Autodesk Fusion 360 part; units mm, degrees
sketch "Sketch1" plane through (0, 0, 0) normal (0, 0, 1) x (1, 0, 0)
  circle A0 centre (0, 0) radius 5
  circle A1 centre (0, 0) radius 2.5
  dimension "d1" = 10
  dimension "d2" = 5
extrude "Extrude1" add sketch "Sketch1" along normal blind 10
sketch "Sketch2" plane through (0, 0, 10) normal (0, 0, 1) x (-1, 0, 0)
  circle A0 centre (0, 0) radius 2.5
  circle A1 centre (0, 0) radius 5
  line L0 (0, 0) -> (-5.75, 0)
  line L1 (-5.75, 0) -> (-5.75, -5.75)
  line L2 (-5.75, -5.75) -> (5.75, -5.75)
  line L3 (5.75, -5.75) -> (5.75, 5.75)
  line L4 (5.75, 5.75) -> (-5.75, 5.75)
  line L5 (-5.75, 5.75) -> (-5.75, -5.75)
  dimension "d5" = 5.75
  dimension "d6" = 5.75
  dimension "d7" = 11.5
  dimension "d8" = 11.5
extrude "Extrude2" add sketch "Sketch2" along normal blind 13 contours A0 | A1 | L1 L2 L3 L4 L5
fillet "Fillet1" radius 5.75 2 edges at (0, -5.75, 23) (0, 5.75, 23)
hole "Hole1" at (5.75, 0, 17.25) direction (-1, 0, 0) diameter 4 depth 11.5 tip angle 180
equation "d5 = ( 11.5 / 2 ) * 1 mm"
Geometry: final body of the model. Coordinates: model frame, mm. A direction names the side the tool comes from. Coordinates: 2 decimals unless noted, no trailing zeros. Order: outer loops, then holes, each group sorted by start corner. A loop starts at its lowest first (then second) coordinate and runs counter-clockwise, first axis right, second up.
(1) Section query B-B (z = 16). Return the cut outline in (x, y), plus the area to 3 significant figures.
(2) Draft query along Y for faces 3 (the face through (0, 0, 10)), 4 (the face through (-1.08, 4.88, 4.93)), 5 (the face through (-5.75, 0, 15)). Return one class per face: pulls with the +Y half, pulls with the -Y half, needs draft (parallel to the pull), parting line crosses it, or undercut.
(3) Material intervals for probe 1 along Y at (x, z) = (1.5, 17.25); probe 2 along Y at (x, z) = (0, 3); probe 3 along Z at (x, y) = (-2, 0), sorted ascending.
(4) Access query for faces 1 (the face through (-0.54, 2.44, 4.93)), 2 (the face through (0.08, -4.02, 21.36)). Directions: +Z, -Z, +X, -X, +Y, -Y. A direction counts if a zero-diameter tool reaches every point of the face in a straight line with its end or side. Return the directions, or none.
(5) Section query D-D (z = 9.5). Return the cut outline in (x, y).
(6) First-contact query: pin 1 (3 mm diameter, centred on x = -1.5, y = -4.5, fed in from +Z); pin 2 (3 mm diameter, centred on x = 1.5, y = -2, fed in from +Z); pin 3 (4.5 mm diameter, centred on x = 0, y = 0, fed in from -Z). Flat tips, straight axial feed; report the tip coordinate or a pass-through.
(7) Section query A-A (y = -1). Return the cut outline in (x, z).
Solution:
1. outline: (-5.75, -5.75) - (5.75, -5.75) - (5.75, -1.56) - (-5.75, -1.56) - close; (-5.75, 1.56) - (5.75, 1.56) - (5.75, 5.75) - (-5.75, 5.75) - close
1. area: 96.3 mm2
2. face 3: undercut
2. face 4: parting line crosses it
2. face 5: needs draft
3. probe 1: y = -5.75 to -2, 2 to 5.75
3. probe 2: y = -5 to -2.5, 2.5 to 5
3. probe 3: z = 10 to 15.25, 19.25 to 23
4. face 1: -Z
4. face 2: +Z, +X, -X, -Y
5. outline: circle Ø10 at (0, 0); hole circle Ø5 at (0, 0)
6. pin 1: stops at z = 22.16
6. pin 2: stops at z = 22.98
6. pin 3: stops at z = 10
7. outline: (-5.75, 10) - (-4.9, 10) - (-4.9, 0) - (-2.29, 0) - (-2.29, 10) - (2.29, 10) - (2.29, 0) - (4.9, 0) - (4.9, 10) - (5.75, 10) - (5.75, 15.52) - (-5.75, 15.52) - close; (-5.75, 18.98) - (5.75, 18.98) - (5.75, 22.91) - (-5.75, 22.91) - close
